The listing builds one solid part. Answer for the finished solid, in the listing's coordinates (mm). A direction names the side the tool comes from. Round coordinates to 2 decimals unless told otherwise and drop trailing zeros. Write each loop counter-clockwise with the first axis right and the second up, starting at its lowest first coordinate (ties: lowest second). Pieces come first, ordered by that corner, then holes. Notation, with made-up numbers: (68.5, 30) - (93.5, 30) arc R15 ccw to (93.5, 38) - close; hole circle Ø11 at (-35.75, -23). An arc over 180 degrees is marked (long way). Use a Markdown table: item, result. Add a question column.
1) Determine the mould class of faces 1 (the flat face through (0, 0, 0)), 2 (the cylindrical face through (10.965, 5.685, -1.083)), 3 (the flat face through (8, 3, -3.994)) for opening direction Z: +Z half, -Z half, draft (parallel to the pull), parting line (faces both ways), or undercut.
2) A cutting plane is placed at D-D (x = 9.25). Give the vertices of the cut face in (y, z).
3) A cutting plane is placed at B-B (x = -4.5). Give the vertices of the cut face in (y, z), then the cut area to 3 significant figures.
4) Find the intervals of material crossed by probe 1 along X at (y, z) = (3.25, -2.25); probe 2 along Y at (x, z) = (-1, -2.75); probe 3 along X at (y, z) = (1.25, 1.5), in increasing order. Write a range as from..to.
5) A tool of negligible diameter and unlimited length cuts with its end or side. For faces 4 (the flat face through (0, 1, 0)), 5 (the cylindrical face through (10.965, 5.787, 2.055)), 6 (the flat face through (2.8, 0.6, 4)), from which of +Z, -Z, +X, -X, +Y, -Y can it reach the whole face along a straight path? Write none if from no direction.
6) This flat-tipped pin is pushed along its axis until it touches: P1, Ø2, axis at x = -3.5, z = -2.5, coming from the +Y side. Where does it stop, or does it pass through?
7) A cutting plane is placed at C-C (y = 2). Give the vertices of the cut face in (x, z).
8) A cutting plane is placed at A-A (z = 1.5). Give the vertices of the cut face in (x, y), then the cut area to 3 significant figures.
```python
from build123d import *

# Parameters (mm, degrees)
SKETCH1_W           = 15
SKETCH1_H           = 8
BOSS_EXTRUDE1_DEPTH = 1
SKETCH2_W           = 7.993829057
SKETCH2_H           = 7
BOSS_EXTRUDE2_DEPTH = 1
SKETCH3_R           = 1.444324147
SKETCH3_R_2         = 1.5
BOSS_EXTRUDE3_DEPTH = 5


with BuildPart() as part:
    # Sketch1 → Boss-Extrude1 (new body)
    with BuildSketch(Plane(origin=(0, 0, 0), x_dir=(1, 0, 0), z_dir=(0, 1, 0))):
        Rectangle(SKETCH1_W, SKETCH1_H)
    extrude(amount=BOSS_EXTRUDE1_DEPTH)

    # Sketch2 → Boss-Extrude2 (add)
    with BuildSketch(Plane(origin=(7.5, 0, 0), x_dir=(0, 0, -1), z_dir=(1, 0, 0))):
        with Locations((-0.003085471, 3.5)):
            Rectangle(SKETCH2_W, SKETCH2_H)
    extrude(amount=BOSS_EXTRUDE2_DEPTH)

    # Sketch3 → Boss-Extrude3 (add)
    with BuildSketch(Plane(origin=(8.5, 0, 0), x_dir=(0, 0, -1), z_dir=(1, 0, 0))):
        with Locations((-1.866576137, 4.354733514)):
            Circle(SKETCH3_R)
        with Locations(Location((1.775399333, 4.354733514, 0), (0, 0, 180))):
            Circle(SKETCH3_R_2)
    extrude(amount=BOSS_EXTRUDE3_DEPTH)


solid = part.part
```
Entries:
| question | item | result |
|---|---|---|
| 1 | face 1 | draft |
| 1 | face 2 | undercut |
| 1 | face 3 | -Z half |
| 2 | outline | circle Ø3 at (4.35, -1.78); circle Ø2.89 at (4.35, 1.87) |
| 3 | outline | (0, -4) - (1, -4) - (1, 4) - (0, 4) - close |
| 3 | area | 8.00 mm² |
| 4 | probe 1 | x = 7.5..13.5 |
| 4 | probe 2 | y = 0..1 |
| 4 | probe 3 | x = 7.5..8.5 |
| 5 | face 4 | +Z, -Z, -X, +Y |
| 5 | face 5 | +X |
| 5 | face 6 | +Z, +X, -X, +Y, -Y |
| 6 | P1 | stops at y = 1 |
| 7 | outline | (7.5, -3.99) - (8.5, -3.99) - (8.5, 4) - (7.5, 4) - close |
| 8 | outline | (-7.5, 0) - (8.5, 0) - (8.5, 2.96) - (13.5, 2.96) - (13.5, 5.75) - (8.5, 5.75) - (8.5, 7) - (7.5, 7) - (7.5, 1) - (-7.5, 1) - close |
| 8 | area | 36.0 mm² |
